```python
from build123d import *

# Parameters (mm, degrees)
CROQUIS1_R              = 15
SALIENTE_EXTRUIR1_DEPTH = 100
CROQUIS2_R              = 15


with BuildPart() as part:
    # Croquis1 → Saliente-Extruir1 (new body)
    with BuildSketch(Plane(origin=(0, 0, 0), x_dir=(1, 0, 0), z_dir=(0, 1, 0))):
        with Locations(Location((0, 0, 0), (0, 0, 270))):
            Circle(CROQUIS1_R)
    extrude(amount=-SALIENTE_EXTRUIR1_DEPTH)

    # Barrer1: sweep along a curve in space
    with BuildLine() as barrer1_path:
        Line((0, -100, 0), (0, -955, 0))
        ThreePointArc((0, -955, 0), (0, -986.819805153, 13.180194847), (0, -1000, 45))
        Line((0, -1000, 45), (0, -1000, 1555))
        ThreePointArc((0, -1000, 1555), (0, -1013.180194847, 1586.819805153), (0, -1045, 1600))
        Line((0, -1045, 1600), (0, -1200, 1600))
    # Croquis2 → Barrer1 (sweep)
    with BuildSketch(Plane.XZ.offset(100)):
        Circle(CROQUIS2_R)
    sweep(path=barrer1_path.line)


solid = part.part
```
CAD build for the part. Positions are in the model's coordinates, mm. Coordinates: 2 decimals unless noted, no trailing zeros. Order: outer loops, then holes, each group sorted by start corner. A loop starts at its lowest first (then second) coordinate and runs counter-clockwise, first axis right, second up. Notation, with made-up numbers: M 64.25,20.25 L 74.25,20.25 A14 ccw 74.25,44.25 Z; hole C 75,75 d7. An arc over 180 degrees is marked long. Answer as CSV lines item,"result".
1) Flat gauge pins, fed straight in: P1, Ø10, axis at x = -6, z = 731, coming from the +Y side; P2, Ø2, axis at x = -4.5, z = 337.5, coming from the +Y side; P3, Ø8, axis at x = -8, z = 591.5, coming from the -Y side. Where does each tip first touch, or does it go through?
Verdict:
P1,"y = -985.03"
P2,"y = -985.41"
P3,"y = -1014.46"
2) Cut at A-A (y = -339.5). List the corners of the cut face in (x, z).
Verdict:
outline,"C 0,0 d30"
3) Drill centre lines: L1, parallel to Y at x = 3, z = 1310.5; L2, parallel to Z at x = -3, y = -556.5; L3, parallel to Z at x = 0.5, y = -262. Where is each one in solid material? Low to high. Write a range as from..to.
Verdict:
L1,"-1014.7..-985.3"
L2,"-14.7..14.7"
L3,"-14.99..14.99"
